Verification items for the finished model (mm, model axes). A direction names the side the tool comes from. Give positions to 0.01 mm unless a question says otherwise; leave off trailing zeros. Loops run counter-clockwise (first coordinate to the right, second up) from the corner with the lowest first, then second, coordinate; pieces in that order, holes last. Notation, with made-up numbers: (26, 44.25) - (71, 44.25) arc R17 ccw to (71, 62.25) - close; hole circle Ø11 at (26.5, 56.25). An arc over 180 degrees is marked (long way). One line per item, written item: value. Start each with the question number.
1. Sectioned sample at A-A (z = 4.4). Record the cut outline in (x, y), plus the area to 3 significant figures.
2. Sectioned sample at C-C (x = 36.5). Record the cut outline in (y, z), plus the area to 3 significant figures.
3. Scan lines: L1, parallel to Y at x = 4, z = 2.75; L2, parallel to X at y = 8, z = 1.5; L3, parallel to Z at x = 38, y = 12.25. Record each from-to range of solid material in increasing order. Write a range as [from, to].
4. Sectioned sample at B-B (y = -2). Record the cut outline in (x, z).
5. Mould release check, pull along Y, two halves, no side actions. Record for faces 4 (the flat face through (-41, 1, 0)), 5 (the flat face through (41, -3.596, 2)): pulls with the +Y half, pulls with the -Y half, needs draft (parallel to the pull), parting line crosses it, or undercut.
6. Sectioned sample at D-D (x = -61). Record the cut outline in (y, z), plus the area to 3 significant figures.
7. Access from +Z, -Z, +X, -X, +Y, -Y to the whole of each face (thin tool, end or side, straight path). Record for faces 1 (the flat face through (51.113, 1, 6)), 2 (the cylindrical face through (65.04, 0.85, 4.85)), 3 (the flat face through (41, 5.427, 2)).
8. Gauge pin test, flat ends, axial feed: pin 1 (4 mm diameter, centred on x = 63.61, z = 4.4, fed in from +Y); pin 2 (1.2 mm diameter, centred on y = 7, z = 2, fed in from +X); pin 3 (2 mm diameter, centred on y = -9.5, z = 1, fed in from +X). Record the tip position at first contact, or that the pin passes through.
from build123d import *

# Parameters (mm, degrees)
F1_DEPTH = 2.8
F2_DEPTH = 23.8
F3_DEPTH = 23.89
F4_DEPTH = 42.8
F5_W     = 23.89
F5_H     = 9.0229478665
F6_DEPTH = 6
F7_R     = 1.5
F8_DEPTH = 9.0229478665
F9_DEPTH = 1.439


with BuildPart() as f1:
    # F0 (on Top) → F1 (new body)
    with BuildSketch(Plane.XY):
        Polygon((-75.0034600496, -12.3867541552), (75.0034600496, -12.3867541552), (75.0034600496, -6.3421353698), (-10.3727839887, -6.3421353698), (-10.3727839887, -3.5960208625), (75.0034600496, -3.5960208625), (75.0034600496, 5.426927004), (-10.3727839887, 5.426927004), (-10.3727839887, 7.7807395719), (75.0034600496, 7.7807395719), (75.0034600496, 12.3867541552), (-75.0034600496, 12.3867541552), align=None)
    extrude(amount=F1_DEPTH)

    # F2 (cut): a face of the model
    f2_faces = [f1.faces().sort_by_distance(p)[0] for p in [
        (75.0034600496, -9.3644447625, 1.4),
    ]]
    extrude(f2_faces, amount=-F2_DEPTH, mode=Mode.SUBTRACT)

    # F3 (cut): a face of the model
    f3_faces = [f1.faces().sort_by_distance(p)[0] for p in [
        (75.0034600496, 10.0837468635, 1.4),
    ]]
    extrude(f3_faces, amount=-F3_DEPTH, mode=Mode.SUBTRACT)

    # F4 (add): a face of the model
    f4_faces = [f1.faces().sort_by_distance(p)[0] for p in [
        (-75.0034600496, 0, 1.4),
    ]]
    extrude(f4_faces, amount=F4_DEPTH)

    # F5 (on face) → F6 (join)
    with BuildSketch(Plane.XY.offset(2.8)):
        with Locations((63.0584600496, 0.9154530708)):
            Rectangle(F5_W, F5_H)
    extrude(amount=F6_DEPTH)

    # F7 (on face) → F8 (cut, through all)
    with BuildSketch(Plane.XZ.offset(3.5960208625)):
        with Locations((63.6097043753, 4.4)):
            Circle(F7_R)
    extrude(amount=-F8_DEPTH, mode=Mode.SUBTRACT)

    # F9 (add): a face of the model
    f9_faces = [f1.faces().sort_by_distance(p)[0] for p in [
        (-33.345, 12.3867541552, 1.4),
    ]]
    extrude(f9_faces, amount=F9_DEPTH)


solid = f1.part
Results are:
1. outline: (51.11, -3.6) - (62.11, -3.6) - (62.11, 5.43) - (51.11, 5.43) - close; (65.11, -3.6) - (75, -3.6) - (75, 5.43) - (65.11, 5.43) - close
1. area: 188 mm^2
2. outline: (-12.39, 0) - (-6.34, 0) - (-6.34, 2.8) - (-12.39, 2.8) - close; (-3.6, 0) - (5.43, 0) - (5.43, 2.8) - (-3.6, 2.8) - close; (7.78, 0) - (13.83, 0) - (13.83, 2.8) - (7.78, 2.8) - close
2. area: 59.1 mm^2
3. L1: y = [-12.39, -6.34], [-3.6, 5.43], [7.78, 13.83]
3. L2: x = [-117.8, 51.11]
3. L3: z = [0, 2.8]
4. outline: (-117.8, 0) - (75, 0) - (75, 8.8) - (51.11, 8.8) - (51.11, 2.8) - (-117.8, 2.8) - close; hole circle Ø3 at (63.61, 4.4)
5. face 4: needs draft
5. face 5: undercut
6. outline: (-12.39, 0) - (13.83, 0) - (13.83, 2.8) - (-12.39, 2.8) - close
6. area: 73.4 mm^2
7. face 1: +Z, -X, +Y, -Y
7. face 2: +Y, -Y
7. face 3: +Z, -Z, +X
8. pin 1: stops at y = 5.43
8. pin 2: stops at x = -10.37
8. pin 3: stops at x = 51.2
